Autodesk Inventor part; units mm, degrees
ref_plane "YZ Plane" through (0, 0, 0) normal (1, 0, 0) x (0, 1, 0)
ref_plane "XZ Plane" through (0, 0, 0) normal (0, 1, 0) x (-1, 0, 0)
ref_plane "XY Plane" through (0, 0, 0) normal (0, 0, 1) x (1, 0, 0)
sketch "Sketch1" plane through (0, 0, 0) normal (0, 0, 1) x (1, 0, 0)
  line L0 (-21, -21) -> (21, -21)
  line L1 (21, -21) -> (21, 21)
  line L2 (21, 21) -> (-21, 21)
  line L3 (-21, 21) -> (-21, -21)
  line L4 (-21, -21) -> (21, 21) construction
  line L5 (21, -21) -> (-21, 21) construction
  line L6 (-18, -18) -> (18, -18)
  line L7 (18, -18) -> (18, 18)
  line L8 (18, 18) -> (-18, 18)
  line L9 (-18, 18) -> (-18, -18)
  line L10 (-18, -18) -> (18, 18) construction
  line L11 (18, -18) -> (-18, 18) construction
  line L12 (18, 18) -> (13.26, 18)
  line L13 (13.26, 18) -> (13.26, 13.26)
  line L14 (13.26, 13.26) -> (18, 13.26)
  line L15 (18, 13.26) -> (18, 18)
  line L16 (18, 18) -> (14.885, 18)
  line L17 (14.885, 18) -> (14.885, 14.885)
  line L18 (14.885, 14.885) -> (18, 14.885)
  line L19 (18, 14.885) -> (18, 18)
  circle A0 centre (14.885, 14.885) radius 1.625
  line L20 (18, 18) -> (11.3, 18)
  line L21 (11.3, 18) -> (11.3, 11.3)
  line L22 (11.3, 11.3) -> (18, 11.3)
  line L23 (18, 11.3) -> (18, 18)
  circle A1 centre (13.26, 13.26) radius 1.96
  point P0 (0, 0)
  dimension "d0" = 42
  dimension "d1" = 42
  dimension "d2" = 36
  dimension "d3" = 36
  dimension "d4" = 4.74
  dimension "d5" = 4.74
  dimension "d6" = 3.115
  dimension "d7" = 6.7
  dimension "d8" = 6.7
extrude "Extrusion1" add sketch "Sketch1" along normal blind 2 contours L3 L2 L1 L0 | L22 A1 L14 L7 | L8 L13 A1 L21 | L14 A1 A0 L18 L7 | L22 L21 A1 | A1 L13 L14 | L8 L17 A0 A1 L13 | L18 A0 L17 L8 L7 | L14 A0 A1 | A1 A0 L13 | A0 A1 L17 L18 | L18 L17 A0 | L14 L13 A0 | A0 A1
mirror "Mirror1" about plane through (0, 0, 0) normal (1, 0, 0) of "Extrusion1"
mirror "Mirror2" about plane through (0, 0, 0) normal (0, 1, 0) of "Extrusion1", "Mirror1"
fillet "Fillet1" radius 2.25 4 edges at (-11.3, 11.3, 1) (11.3, 11.3, 1) (11.3, -11.3, 1) (-11.3, -11.3, 1)
sketch "Sketch2" plane through (0, 0, 2) normal (0, 0, 1) x (1, 0, 0)
  line L0 (21, -21) -> (21, 21)
  line L1 (21, 21) -> (14.885, 21)
  line L2 (14.885, 21) -> (14.885, 14.885)
  line L3 (14.885, 14.885) -> (21, 14.885)
  line L4 (21, 14.885) -> (21, 21)
  circle A0 centre (14.885, 14.885) radius 1.625
  point P0 (0, 0)
  dimension "d12" = 6.115
  dimension "d13" = 6.115
  dimension "d14" = 3.25
extrude "Extrusion2" cut sketch "Sketch2" against normal blind 2 contours A0 L2 L3 | L3 L2 A0
mirror "Mirror3" about plane through (0, 0, 0) normal (0, 1, 0) of "Extrusion2"
mirror "Mirror4" about plane through (0, 0, 0) normal (1, 0, 0) of "Extrusion2", "Mirror3"
sketch "Sketch3" plane through (0, 0, 2) normal (0, 0, 1) x (1, 0, 0)
  line L0 (-18, -18) -> (18, -18)
  line L1 (18, -18) -> (18, 18)
  line L2 (18, 18) -> (-18, 18)
  line L3 (-18, 18) -> (-18, -18)
  line L4 (-18, -18) -> (18, 18) construction
  line L5 (18, -18) -> (-18, 18) construction
  line L6 (21, 21) -> (-21, 21)
  line L7 (-21, -21) -> (21, -21)
  line L8 (21, -21) -> (21, 21)
  line L9 (21, 21) -> (-21, 21)
  line L10 (-21, 21) -> (-21, -21)
  line L11 (-21, -21) -> (21, 21) construction
  line L12 (21, -21) -> (-21, 21) construction
  point P0 (0, 0)
  dimension "d17" = 36
  dimension "d18" = 36
extrude "Extrusion3" add sketch "Sketch3" along normal blind 22
sketch "Sketch4" plane through (0, 0, 24) normal (0, 0, 1) x (1, 0, 0)
  line L0 (21, 21) -> (-21, 21)
  line L1 (-21, -21) -> (21, -21)
  line L2 (21, -21) -> (21, 21)
  line L3 (21, 21) -> (-21, 21)
  line L4 (-21, 21) -> (-21, -21)
  line L5 (-21, -21) -> (21, 21) construction
  line L6 (21, -21) -> (-21, 21) construction
  line L7 (-19.7, -19.7) -> (19.7, -19.7)
  line L8 (19.7, -19.7) -> (19.7, 19.7)
  line L9 (19.7, 19.7) -> (-19.7, 19.7)
  line L10 (-19.7, 19.7) -> (-19.7, -19.7)
  line L11 (-19.7, -19.7) -> (19.7, 19.7) construction
  line L12 (19.7, -19.7) -> (-19.7, 19.7) construction
  point P0 (0, 0)
  dimension "d21" = 39.4
  dimension "d22" = 39.4
extrude "Extrusion4" add sketch "Sketch4" along normal blind 3
fillet "Fillet2" radius 2 4 edges at (21, -21, 13.5) (21, 21, 13.5) (-21, 21, 13.5) (-21, -21, 13.5)
properties part number "camerashield"
The model under review builds one solid part; all positions refer to its coordinate system, in mm. A direction names the side the tool comes from. Round coordinates to 2 decimals unless told otherwise and drop trailing zeros. Loops run counter-clockwise (first coordinate to the right, second up) from the corner with the lowest first, then second, coordinate; pieces in that order, holes last. Notation, with made-up numbers: (-4, 23) -> (52, 23) arc R25 ccw to (52, 53) -> close; hole circle Ø6 at (34.25, 68.25). An arc over 180 degrees is marked (long way). Answer as a JSON object with one key per item and string values. Group by question number.
1) For pin 1 Ø10 at (x, y) = (7, -8.5) entering from -Z; pin 2 Ø5 at (x, y) = (14.885, -14.885) entering from -Z; pin 3 Ø2 at (x, y) = (13.5, 14.5) entering from +Z, all flat-tipped, find the tip position at first contact; note any pin that passes through.
2) For faces 3 (the face through (15, -13, 2)), 4 (the face through (-2, -20, 27)), 5 (the face through (11.94, 11.98, 1.01)), list the 3-axis set-ups (+Z, -Z, +X, -X, +Y, -Y) from which the entire face can be reached by the end or side of a thin tool; tool diameter is ignored.
3) For line 1 (Y direction, x = -13, z = 6); line 2 (X direction, y = -11, z = 25.5), list the stretches that pass through material, from the lowest coordinate up. Write a range as [from, to].
4) Mouldability with a two-part tool opening along Y and no side actions: class faces 1 (the face through (21, 0, 13)), 2 (the face through (11.98, -11.94, 1.01)) as released by +Y, released by -Y, zero draft, split by the parting line, or undercut.
5) We need section A-A on y = 2.5. Write out the cut boundary in (x, z).
6) We need section C-C on z = 21. Write out the cut boundary in (x, y), then the cut area to 3 significant figures.
Result set:
{
 "1": {"pin 1": "through", "pin 2": "z = 0", "pin 3": "z = 2"},
 "2": {"face 3": "+Z", "face 4": "+Z, +X, -X, +Y, -Y", "face 5": "+Z, -Z"},
 "3": {"line 1": "[-21, -18], [18, 21]", "line 2": "[-21, -19.7], [19.7, 21]"},
 "4": {"face 1": "zero draft", "face 2": "undercut"},
 "5": {"outline": "(-21, 0) -> (-18, 0) -> (-18, 24) -> (-19.7, 24) -> (-19.7, 27) -> (-21, 27) -> close; (18, 0) -> (21, 0) -> (21, 27) -> (19.7, 27) -> (19.7, 24) -> (18, 24) -> close"},
 "6": {"outline": "(-21, -19) arc R2 ccw to (-19, -21) -> (19, -21) arc R2 ccw to (21, -19) -> (21, 19) arc R2 ccw to (19, 21) -> (-19, 21) arc R2 ccw to (-21, 19) -> close; hole (-18, -18) -> (18, -18) -> (18, 18) -> (-18, 18) -> close", "area": "465 mm²"}
}
